from build123d import *

# Parameters (mm, degrees)
SKETCH1_R           = 1.5
BOSS_EXTRUDE1_DEPTH = 3.05
CUT_EXTRUDE1_DEPTH  = 67.231469106


with BuildPart() as part:
    # Sketch1 → Boss-Extrude1 (new body)
    with BuildSketch(Plane(origin=(0, 0, 0), x_dir=(1, 0, 0), z_dir=(0, 1, 0))):
        Polygon((3.05, 20.05), (3.05, 12), (0, 12), (0, 4), (3.05, 4), (3.05, 0), (63.05, 0), (63.05, 4), (66.1, 4), (66.1, 12), (63.05, 12), (63.05, 20.05), align=None)
        with Locations(Location((54.05, 7, 0), (0, 0, 270))):
            Circle(SKETCH1_R, mode=Mode.SUBTRACT)
        with Locations(Location((12.05, 7, 0), (0, 0, 270))):
            Circle(SKETCH1_R, mode=Mode.SUBTRACT)
    extrude(amount=BOSS_EXTRUDE1_DEPTH)

    # Sketch5 → CSK for M3 Flat Head Machine Screw1 (revolve, cut)
    with BuildSketch(Plane(origin=(12.05, 3.05, -7), x_dir=(0, 0, 1), z_dir=(1, 0, 0))):
        Polygon((0, 0), (0, 3.05), (1.6, 3.05), (1.6, 1.55), (3.15, 0), align=None)
    revolve(axis=Axis((12.05, 9.4, -7), (0, -1, 0)), mode=Mode.SUBTRACT)

    # Sketch7 → CSK for M3 Flat Head Machine Screw2 (revolve, cut)
    with BuildSketch(Plane(origin=(54.05, 3.05, -7), x_dir=(0, 0, 1), z_dir=(1, 0, 0))):
        Polygon((0, 0), (0, 3.05), (1.6, 3.05), (1.6, 1.55), (3.15, 0), align=None)
    revolve(axis=Axis((54.05, 9.4, -7), (0, -1, 0)), mode=Mode.SUBTRACT)

    # Sketch8 → Cut-Extrude1 (cut, through all)
    with BuildSketch(Plane(origin=(63.05, 0, 0), x_dir=(0, 0, -1), z_dir=(1, 0, 0))):
        Polygon((20.05, 3.05), (17, 0), (20.05, 0), align=None)
    extrude(amount=-CUT_EXTRUDE1_DEPTH, mode=Mode.SUBTRACT)


solid = part.part
CAD build for the part. Positions are in the model's coordinates, mm. A direction names the side the tool comes from. Coordinates: 2 decimals unless noted, no trailing zeros. Write each loop counter-clockwise with the first axis right and the second up, starting at its lowest first coordinate (ties: lowest second). Pieces come first, ordered by that corner, then holes. Notation, with made-up numbers: M 10,64 L 39,64 A30 cw 39,100 Z; hole C 79,84 d4. An arc over 180 degrees is marked long. Answer as a JSON object with one key per item and string values. Group by question number.
1) Pin check, flat tips, straight feed: pin 1 Ø5 at (x, z) = (58.5, -8.5) entering from -Y; pin 2 Ø1.5 at (x, y) = (64.5, 1) entering from +Z; pin 3 Ø1.5 at (x, y) = (2, 1) entering from -Z; pin 4 Ø1.5 at (y, z) = (2, -2.5) entering from +X. Stop position of each tip, or through.
2) Saw through at A-A (y = 2). Write the cut outline in (x, z), plus the area to 3 significant figures.
3) Wall check: line 1 (X direction, y = 0.85, z = -7); line 2 (X direction, y = 2.55, z = -8.25); line 3 (X direction, y = 1, z = -15). Give the ranges that are in metal, low to high. Write a range as from..to.
4) Saw through at D-D (x = 23). Write the cut outline in (y, z), plus the area to 3 significant figures.
5) Tool access for faces 1 (the face through (33, 0, -9)), 2 (the face through (65, 2, -4)), 3 (the face through (3.05, 2, -15)), 4 (the face through (2, 2, -4)), 5 (the face through (63.05, 2, -15)): list every direction of +Z, -Z, +X, -X, +Y, -Y with a clear straight run to the whole face (end or side of a thin tool).
6) Saw through at C-C (z = -13.75). Write the cut outline in (x, y).
7) Saw through at B-B (x = 54.05). Write the cut outline in (y, z), plus the area to 3 significant figures.
Values follow:
{
 "1": {"pin 1": "stops at y = 0", "pin 2": "stops at z = -4", "pin 3": "stops at z = -12", "pin 4": "stops at x = 63.05"},
 "2": {"outline": "M 0,-12 L 3.05,-12 L 3.05,-19 L 63.05,-19 L 63.05,-12 L 66.1,-12 L 66.1,-4 L 63.05,-4 L 63.05,0 L 3.05,0 L 3.05,-4 L 0,-4 Z; hole C 12.05,-7 d4.2; hole C 54.05,-7 d4.2", "area": "1,160 mm2"},
 "3": {"line 1": "x = 0..10.45, 13.65..52.45, 55.65..66.1", "line 2": "x = 0..9.71, 14.39..51.71, 56.39..66.1", "line 3": "x = 3.05..63.05"},
 "4": {"outline": "M 0,-17 L 3.05,-20.05 L 3.05,0 L 0,0 Z", "area": "56.5 mm2"},
 "5": {"face 1": "+Z, -Z, +X, -X, -Y", "face 2": "+Z, +X, +Y, -Y", "face 3": "-Z, -X, +Y, -Y", "face 4": "+Z, -X, +Y, -Y", "face 5": "-Z, +X, +Y, -Y"},
 "6": {"outline": "M 3.05,0 L 63.05,0 L 63.05,3.05 L 3.05,3.05 Z"},
 "7": {"outline": "M 0,-17 L 3.05,-20.05 L 3.05,-10.15 L 1.5,-8.6 L 0,-8.6 Z; M 0,-5.4 L 1.5,-5.4 L 3.05,-3.85 L 3.05,0 L 0,0 Z", "area": "44.3 mm2"}
}
